from build123d import *

# Parameters (mm, degrees)
F1_DEPTH       = 25
F4_D           = 3.3
F4_CBORE_D     = 6.1
F4_CBORE_DEPTH = 4
F3_R           = 1.5
F5_DEPTH       = 3
F6_DEPTH       = 3
F9_DEPTH       = 4


with BuildPart() as f1:
    # F0 (on Top) → F1 (new body)
    with BuildSketch(Plane.XY):
        with BuildLine():
            ThreePointArc((-0.5, -2.44949), (-1.581139, 1.936492), (2.5, 0))
            ThreePointArc((2.5, 0), (1.936492, -1.581139), (0.5, -2.44949))
            Line((0.5, -2.44949), (0.5, -7.483315))
            ThreePointArc((0.5, -7.483315), (5.477226, -5.123475), (7.5, 0))
            ThreePointArc((7.5, 0), (-5.123475, 5.477226), (-0.5, -7.483315))
            Line((-0.5, -7.483315), (-0.5, -2.44949))
        make_face()
    extrude(amount=F1_DEPTH)

    # F4 (through all)
    with Locations(Plane.YZ.offset(7.5)):
        with Locations((-4.5, 20), (-4.5, 5)):
            CounterBoreHole(F4_D / 2, F4_CBORE_D / 2, F4_CBORE_DEPTH)

    # F3 (on plane+point) → F5 (cut)
    with BuildSketch(Plane.YZ.offset(7.5)):
        with Locations((-4.5, 5)):
            Circle(F3_R)
    extrude(amount=-F5_DEPTH, mode=Mode.SUBTRACT)

    # F3 (on plane+point) → F6 (cut)
    with BuildSketch(Plane.YZ.offset(7.5)):
        with Locations((-4.5, 20)):
            Circle(F3_R)
    extrude(amount=-F6_DEPTH, mode=Mode.SUBTRACT)

    # F8 (on plane+point) → F9 (cut)
    with BuildSketch(Plane.YZ.offset(-7.5)):
        Polygon((-7.141377, 3.475), (-4.5, 1.95), (-1.858623, 3.475), (-1.858623, 6.525), (-4.5, 8.05), (-7.141377, 6.525), align=None)
        Polygon((-1.858623, 18.475), (-1.858623, 21.525), (-4.5, 23.05), (-7.141377, 21.525), (-7.141377, 18.475), (-4.5, 16.95), align=None)
    extrude(amount=F9_DEPTH, mode=Mode.SUBTRACT)


solid = f1.part
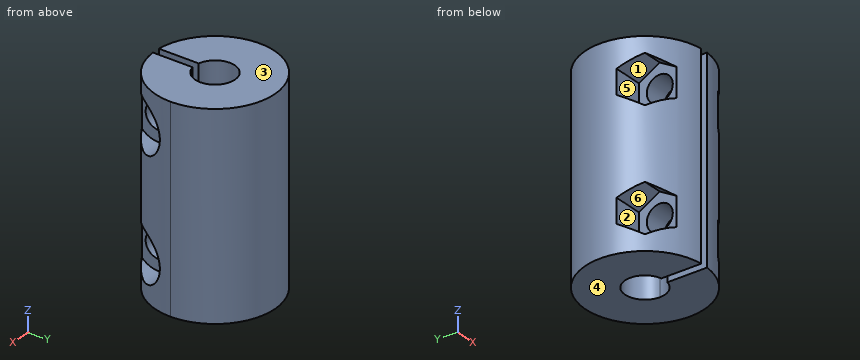
Here's how the part is built. I have some questions about the finished solid (model axes, mm). Face numbers are marked on the shaded views. A direction names the side the tool comes from. Round coordinates to 2 decimals unless told otherwise and drop trailing zeros. Loops run counter-clockwise (first coordinate to the right, second up) from the corner with the lowest first, then second, coordinate; pieces in that order, holes last. Notation, with made-up numbers: (21.25, 71.5) -> (27.25, 71.5) arc R6 cw to (27.25, 75.5) -> close; hole circle Ø6 at (-27.5, 22). An arc over 180 degrees is marked (long way). Write each question's results on one line, items separated by ' | '.
(1) If I drill on L1, parallel to Z at x = 4.9, y = -4.5; L2, parallel to Z at x = -1.6, y = -4.5; L3, parallel to X at y = -6, z = 18, over which ranges is the centre line in solid material (lowest first)?
Worked answers:
L1: 0 to 1.95, 8.05 to 16.95, 23.05 to 25 | L2: 0 to 3.35, 6.65 to 18.35, 21.65 to 25 | L3: -3.5 to -0.5, 0.5 to 3.5
(2) For P1, Ø2, axis at y = -3, z = 19.5, coming from the +X side; P2, Ø5.5, axis at y = -4, z = 21, coming from the -X side; P3, Ø4, axis at y = -5.5, z = 8.5, coming from the +X side; P4, Ø1.5, axis at y = 0.5, z = 7.5, coming from the +X side, each with a flat end and sliding along its axis, tell me the tip position at first contact or that it passes through.
Worked answers:
P1: x = 3.5 | P2: x = -7.4 | P3: x = 6.63 | P4: x = 7.5
(3) For the marked faces 4, 5 and 6, which set-ups out of +Z, -Z, +X, -X, +Y, -Y let a thin tool reach every point of the face, with its end or its side?
Worked answers:
face 4: -Z, +X, -X, +Y, -Y | face 5: -X, -Y | face 6: -X
(4) If we section it at C-C, the plane y = 1.75: List the corners of the cut face in (x, z) for me.
Worked answers:
outline: (-7.29, 0) -> (-1.79, 0) -> (-1.79, 25) -> (-7.29, 25) -> close; (1.79, 0) -> (7.29, 0) -> (7.29, 25) -> (1.79, 25) -> close
(5) If we section it at D-D, the plane x = 5.5: List the corners of the cut face in (y, z) for me, then the cut area to 3 significant figures.
Worked answers:
outline: (-5.1, 0) -> (5.1, 0) -> (5.1, 25) -> (-5.1, 25) -> (-5.1, 22.99) arc R3.05 cw (long way) to (-5.1, 17.01) -> (-5.1, 7.99) arc R3.05 cw (long way) to (-5.1, 2.01) -> close | area: 218 mm2
(6) We'd pull the mould along Y, two halves only. Please class the marked faces 1, 2 and 3: released by +Y, released by -Y, zero draft, split by the parting line, or undercut.
Worked answers:
face 1: undercut | face 2: released by -Y | face 3: zero draft
(7) If we section it at B-B, the plane z = 5: List the corners of the cut face in (x, y) for me, then the cut area to 3 significant figures.
Worked answers:
outline: (-7.27, -1.86) -> (-3.5, -1.86) -> (-3.5, -2.85) -> (-0.5, -2.85) -> (-0.5, -2.45) arc R2.5 cw (long way) to (0.5, -2.45) -> (0.5, -2.85) -> (3.5, -2.85) -> (3.5, -1.45) -> (7.36, -1.45) arc R7.5 ccw (long way) to start; (-3.5, -6.63) arc R7.5 ccw to (-0.5, -7.48) -> (-0.5, -6.15) -> (-3.5, -6.15) -> close; (0.5, -7.48) arc R7.5 ccw to (3.5, -6.63) -> (3.5, -6.15) -> (0.5, -6.15) -> close | area: 107 mm2
(8) If we section it at A-A, the plane x = -2: List the corners of the cut face in (y, z) for me.
Worked answers:
outline: (-7.23, 0) -> (-1.5, 0) -> (-1.5, 25) -> (-7.23, 25) -> close; (1.5, 0) -> (7.23, 0) -> (7.23, 25) -> (1.5, 25) -> close; hole circle Ø3.3 at (-4.5, 5); hole circle Ø3.3 at (-4.5, 20)
